Could you check a few things on this model? Use its own coordinates, in mm. A direction names the side the tool comes from. Give positions to 0.01 mm unless a question says otherwise; leave off trailing zeros. Order: outer loops, then holes, each group sorted by start corner. A loop starts at its lowest first (then second) coordinate and runs counter-clockwise, first axis right, second up. Notation, with made-up numbers: (47, 56) -> (62, 56) arc R30 ccw to (62, 81) -> close; hole circle Ø10 at (-10, -38.5). An arc over 180 degrees is marked (long way). Write each question's results on one line, items separated by ' | '.
```python
from build123d import *

# Parameters (mm, degrees)
BOSS_EXTRUDE1_DEPTH   = 57.15
SKETCH2_W             = 22.86
SKETCH2_H             = 3.683
BOSS_EXTRUDE2_DEPTH   = 24.13
SKETCH3_R             = 3.048
CUT_EXTRUDE1_DEPTH    = 2.54
F_3_0MM_DOWEL_HOLE1_D = 3
SKETCH6_W             = 12.7
SKETCH6_H             = 76.2
CUT_EXTRUDE2_DEPTH    = 6.35
CUT_EXTRUDE3_DEPTH    = 5.08
SKETCH7_R             = 2.54
CUT_EXTRUDE4_DEPTH    = 6.35
CUT_EXTRUDE5_DEPTH    = 76.2


with BuildPart() as part:
    # Sketch1 → Boss-Extrude1 (new body, symmetric)
    with BuildSketch(Plane(origin=(0, 0, 0), x_dir=(1, 0, 0), z_dir=(0, 1, 0))):
        with BuildLine():
            ThreePointArc((30.247337007, 9.652), (0, 31.75), (-30.247337007, 9.652))
            Line((-30.247337007, 9.652), (30.247337007, 9.652))
        make_face()
    extrude(amount=BOSS_EXTRUDE1_DEPTH, both=True)

    # Sketch2 → Boss-Extrude2 (add)
    with BuildSketch(Plane.XZ.offset(57.15)):
        with Locations((0, -11.4935)):
            Rectangle(SKETCH2_W, SKETCH2_H)
    extrude(amount=BOSS_EXTRUDE2_DEPTH)

    # Sketch3 → Cut-Extrude1 (cut)
    with BuildSketch(Plane.XY.offset(-9.652)):
        with Locations((0, -63.641247378)):
            Circle(SKETCH3_R)
        with Locations((-7.62, -76.839474532)):
            Circle(SKETCH3_R)
        with Locations((7.62, -76.839474532)):
            Circle(SKETCH3_R)
    extrude(amount=-CUT_EXTRUDE1_DEPTH, mode=Mode.SUBTRACT)

    # Ø3.0mm Dowel Hole1 (through all)
    with Locations(Plane.XY.offset(-9.652)):
        with Locations((0, -63.641247378), (7.62, -76.839474532), (-7.62, -76.839474532)):
            Hole(F_3_0MM_DOWEL_HOLE1_D / 2)

    # Sketch6 → Cut-Extrude2 (cut)
    with BuildSketch(Plane.XY.offset(-9.652)):
        with Locations((0, 19.05)):
            Rectangle(SKETCH6_W, SKETCH6_H)
    extrude(amount=-CUT_EXTRUDE2_DEPTH, mode=Mode.SUBTRACT)

    # Sketch8 → Cut-Extrude3 (cut)
    with BuildSketch(Plane(origin=(0, 57.15, 0), x_dir=(1, 0, 0), z_dir=(0, 1, 0))):
        with BuildLine():
            Line((2.286933633, 24.02783982), (0, 25.4))
            Line((0, 25.4), (-2.286933633, 24.02783982))
            ThreePointArc((-2.286933633, 24.02783982), (0, 22.733), (2.286933633, 24.02783982))
        make_face()
        with BuildLine():
            Line((-2.286933633, 24.02783982), (0, 25.4))
            Line((0, 25.4), (2.286933633, 24.02783982))
            ThreePointArc((2.286933633, 24.02783982), (2.570227714, 24.688088137), (2.667, 25.4))
            ThreePointArc((2.667, 25.4), (-0.711911863, 27.970227714), (-2.286933633, 24.02783982))
        make_face()
        with BuildLine():
            ThreePointArc((-10.033, 17.78), (-10.129772286, 18.491911863), (-10.413066367, 19.15216018))
            Line((-10.413066367, 19.15216018), (-12.7, 17.78))
            Line((-12.7, 17.78), (-10.033, 17.78))
        make_face()
        with BuildLine():
            Line((-12.7, 17.78), (-10.413066367, 19.15216018))
            ThreePointArc((-10.413066367, 19.15216018), (-15.270227714, 17.068088137), (-10.033, 17.78))
            Line((-10.033, 17.78), (-12.7, 17.78))
        make_face()
        with BuildLine():
            ThreePointArc((15.367, 17.78), (13.411911863, 20.350227714), (10.413066367, 19.15216018))
            Line((10.413066367, 19.15216018), (12.7, 17.78))
            Line((12.7, 17.78), (10.033, 17.78))
            ThreePointArc((10.033, 17.78), (12.7, 15.113), (15.367, 17.78))
        make_face()
        with BuildLine():
            Line((12.7, 17.78), (10.413066367, 19.15216018))
            ThreePointArc((10.413066367, 19.15216018), (10.129772286, 18.491911863), (10.033, 17.78))
            Line((10.033, 17.78), (12.7, 17.78))
        make_face()
    extrude(amount=-CUT_EXTRUDE3_DEPTH, mode=Mode.SUBTRACT)

    # Sketch7 → Cut-Extrude4 (cut)
    with BuildSketch(Plane.XY.offset(-16.002)):
        with Locations((0, 52.07)):
            Circle(SKETCH7_R)
        with Locations((0, 41.91)):
            Circle(SKETCH7_R)
        with Locations((0, 31.75)):
            Circle(SKETCH7_R)
        with Locations((0, 21.59)):
            Circle(SKETCH7_R)
        with Locations((0, 11.43)):
            Circle(SKETCH7_R)
        with Locations((0, 1.27)):
            Circle(SKETCH7_R)
        with Locations((0, -8.89)):
            Circle(SKETCH7_R)
    extrude(amount=-CUT_EXTRUDE4_DEPTH, mode=Mode.SUBTRACT)

    # Sketch9 → Cut-Extrude5 (cut)
    with BuildSketch(Plane(origin=(0, 57.15, 0), x_dir=(1, 0, 0), z_dir=(0, 1, 0))):
        Polygon((6.35, 16.002), (23.796481614, 9.652), (6.35, 9.652), align=None)
        Polygon((-6.35, 16.002), (-23.796481614, 9.652), (-6.35, 9.652), align=None)
    extrude(amount=-CUT_EXTRUDE5_DEPTH, mode=Mode.SUBTRACT)


solid = part.part
```
Q1. Thinking about a two-plate mould opening in X: for faces 5 (the flat face through (-7, -75, -12.192)), 6 (the cylindrical face through (0.561, 0.8, -31.745)), 7 (the flat face through (0, 57.15, -21)), which applies, +X half, -X half, draft (parallel to the pull), parting line (faces both ways), or undercut?
Here are the results:
face 5: undercut | face 6: parting line | face 7: draft
Q2. I'm going to push flat-ended pins straight in: pin 1 Ø3 at (x, y) = (0, 21.59) entering from -Z; pin 2 Ø2.5 at (x, y) = (-7.62, -76.84) entering from -Z; pin 3 Ø5 at (x, y) = (19.5, 30.5) entering from -Z; pin 4 Ø1 at (y, z) = (-29.5, -15.5) entering from +X. Where does each tip first touch, or does it pass through?
Here are the results:
pin 1: stops at z = -31.75 | pin 2: passes through | pin 3: stops at z = -26.82 | pin 4: stops at x = 27.98
Q3. For faces 1 (the flat face through (3, 20, -16.002)), 2 (the cylindrical face through (-0.33, -6.37, -19.13)), 3 (the cylindrical face through (-8.426, -75.575, -12.772)), 4 (the flat face through (0, 52.07, -25)), which set-ups out of +Z, -Z, +X, -X, +Y, -Y let a thin tool reach every point of the face, with its end or its side?
Here are the results:
face 1: +Z, +Y | face 2: +Z | face 3: +Z, -Z | face 4: +Y
Q4. Suppose I cut it at D-D on z = -30.25. Please give me the cut outline in (x, y).
Here are the results:
outline: (-9.64, -57.15) -> (9.64, -57.15) -> (9.64, 57.15) -> (-9.64, 57.15) -> close
Q5. Suppose I cut it at B-B on y = -8.89. Please give me the cut outline in (x, z).
Here are the results:
outline: (-30.25, -9.65) arc R31.75 ccw to (30.25, -9.65) -> (23.8, -9.65) -> (6.35, -16) -> (2.54, -16) -> (2.54, -22.35) -> (-2.54, -22.35) -> (-2.54, -16) -> (-6.35, -16) -> (-23.8, -9.65) -> close
Q6. I need wall thicknesses on line 1 along X through (y, z) = (55.2, -17.78); line 2 along Y through (x, z) = (0, -12.5); line 3 along Z through (x, y) = (-1, -36.5). Which ranges of each line are inside material? Lowest first, please.
Here are the results:
line 1: x = -26.3 to -15.37, -10.03 to 10.03, 15.37 to 26.3 | line 2: y = -81.28 to -65.14, -62.14 to -19.05 | line 3: z = -31.73 to -9.65
Q7. Suppose I cut it at A-A on x = -7.62. Please give me the cut outline in (y, z) (3 decimals).
Here are the results:
outline: (-81.28, -13.335) -> (-78.339, -13.335) -> (-78.339, -12.192) -> (-79.887, -12.192) -> (-79.887, -9.652) -> (-81.28, -9.652) -> close; (-75.339, -13.335) -> (-57.15, -13.335) -> (-57.15, -30.822) -> (57.15, -30.822) -> (57.15, -15.54) -> (-19.05, -15.54) -> (-19.05, -9.652) -> (-73.791, -9.652) -> (-73.791, -12.192) -> (-75.339, -12.192) -> close
Q8. Suppose I cut it at C-C on y = 37. Please give me the cut outline in (x, z).
Here are the results:
outline: (-30.25, -9.65) arc R31.75 ccw to (30.25, -9.65) -> (23.8, -9.65) -> (6.35, -16) -> (-6.35, -16) -> (-23.8, -9.65) -> close
